Part model, mm, in its own coordinate system. Round coordinates to 2 decimals unless told otherwise and drop trailing zeros. Write each loop counter-clockwise with the first axis right and the second up, starting at its lowest first coordinate (ties: lowest second). Pieces come first, ordered by that corner, then holes.
1) Saw through at C-C on y = 4. Write the cut outline in (x, z), and give its area (3 significant figures).
2) Saw through at B-B on x = -20.5. Write the cut outline in (y, z), and give its area (3 significant figures).
3) Flat gauge pins, fed straight in: pin 1 (1.5 mm diameter, centred on x = 63.5, z = 1, fed in from -Y); pin 2 (1.5 mm diameter, centred on y = -6, z = 1, fed in from -X); pin 3 (6 mm diameter, centred on x = 49.5, y = -27.5, fed in from -Z); pin 4 (0.9 mm diameter, centred on y = -40, z = 1.5, fed in from +X). Where does each tip first touch, or does it go through?
4) Drill centre lines: L1, parallel to Y at x = -22, z = 2.4; L2, parallel to Y at x = -3.5, z = 1.7; L3, parallel to X at y = -7, z = 0.75. Where is each one in solid material? Low to high.
5) Saw through at A-A on z = 0.7. Write the cut outline in (x, y), and give its area (3 significant figures).
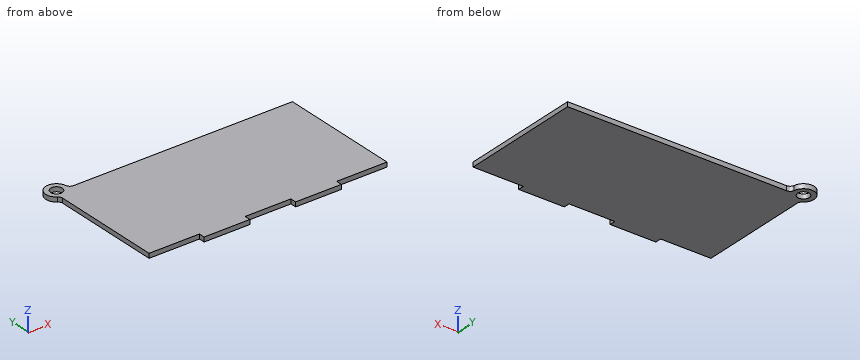
```python
from build123d import *

# Parameters (mm, degrees)
SKETCH1_R           = 3.8
BOSS_EXTRUDE1_DEPTH = 3


with BuildPart() as part:
    # Sketch1 → Boss-Extrude1 (new body)
    with BuildSketch(Plane.XY):
        with BuildLine():
            Line((-45.446220454, -41.816247618), (-45.446220454, -37.816247618))
            Line((-45.446220454, -37.816247618), (-75.446220454, -37.816247618))
            Line((-75.446220454, -37.816247618), (-78.446220454, -37.816247618))
            Line((-78.446220454, -37.816247618), (-78.446220454, 35.332105838))
            ThreePointArc((-78.446220454, 35.332105838), (-78.805197925, 36.755130785), (-79.796220454, 37.837599801))
            ThreePointArc((-79.796220454, 37.837599801), (-79.720698736, 49.578946501), (-69.025418478, 44.733752382))
            ThreePointArc((-69.025418478, 44.733752382), (-68.015121209, 42.908889749), (-66.059360488, 42.183752382))
            Line((-66.059360488, 42.183752382), (77.553779546, 42.183752382))
            Line((77.553779546, 42.183752382), (77.553779546, -37.816247618))
            Line((77.553779546, -37.816247618), (44.553779546, -37.816247618))
            Line((44.553779546, -37.816247618), (44.553779546, -41.816247618))
            Line((44.553779546, -41.816247618), (14.553779546, -41.816247618))
            Line((14.553779546, -41.816247618), (14.553779546, -37.816247618))
            Line((14.553779546, -37.816247618), (-15.446220454, -37.816247618))
            Line((-15.446220454, -37.816247618), (-15.446220454, -41.816247618))
            Line((-15.446220454, -41.816247618), (-45.446220454, -41.816247618))
        make_face()
        with Locations((-75.946220454, 43.683752382)):
            Circle(SKETCH1_R, mode=Mode.SUBTRACT)
    extrude(amount=BOSS_EXTRUDE1_DEPTH)


solid = part.part
```
Completed:
1. outline: (-78.45, 0) - (77.55, 0) - (77.55, 3) - (-78.45, 3) - close
1. area: 468 mm2
2. outline: (-41.82, 0) - (42.18, 0) - (42.18, 3) - (-41.82, 3) - close
2. area: 252 mm2
3. pin 1: stops at y = -37.82
3. pin 2: stops at x = -78.45
3. pin 3: stops at z = 0
3. pin 4: stops at x = 44.55
4. L1: y = -41.82 to 42.18
4. L2: y = -37.82 to 42.18
4. L3: x = -78.45 to 77.55
5. outline: (-79.8, 37.84) arc R3 cw to (-78.45, 35.33) - (-78.45, -37.82) - (-45.45, -37.82) - (-45.45, -41.82) - (-15.45, -41.82) - (-15.45, -37.82) - (14.55, -37.82) - (14.55, -41.82) - (44.55, -41.82) - (44.55, -37.82) - (77.55, -37.82) - (77.55, 42.18) - (-66.06, 42.18) arc R3 cw to (-69.03, 44.73) arc R7 ccw (long way) to start; hole circle Ø7.6 at (-75.95, 43.68)
5. area: 12,800 mm2
